CAD build for the part. Positions are in the model's coordinates, mm. Coordinates: 2 decimals unless noted, no trailing zeros. Order: outer loops, then holes, each group sorted by start corner. A loop starts at its lowest first (then second) coordinate and runs counter-clockwise, first axis right, second up. Notation, with made-up numbers: M -3,33.5 L 19,33.5 A13 cw 19,42.5 Z; hole C 62,29 d1. An arc over 180 degrees is marked long. Write item = value, one per line. Start each with the question number.
```python
from build123d import *

# Parameters (mm, degrees)
SKETCH7_R           = 24
SKETCH7_R_2         = 20.5
BOSS_EXTRUDE6_DEPTH = 3.5
FILLET4_R           = 1.75


with BuildPart() as part:
    # Sketch7 → Boss-Extrude6 (new body)
    with BuildSketch(Plane(origin=(-0.280788986, 0.442554621, -13.906554041), x_dir=(-1, 0, 0), z_dir=(0, 0, -1))):
        with Locations((-13.807967582, -75.62783073)):
            Circle(SKETCH7_R)
        with Locations((-13.807967582, -75.62783073)):
            Circle(SKETCH7_R_2, mode=Mode.SUBTRACT)
    extrude(amount=BOSS_EXTRUDE6_DEPTH)

    # Fillet4
    fillet4_edges = [part.edges().sort_by_distance(p)[0] for p in [
        (37.527178596, -75.18527611, -13.906554041),
        (37.527178596, -75.18527611, -17.406554041),
        (34.027178596, -75.18527611, -13.906554041),
        (34.027178596, -75.18527611, -17.406554041),
    ]]
    fillet(fillet4_edges, radius=FILLET4_R - 0.0001)  # a hair under: the kernel refuses the full size


solid = part.part
```
1. Flat gauge pins, fed straight in: pin 1 (1 mm diameter, centred on y = -75.5, z = -17, fed in from -X); pin 2 (2 mm diameter, centred on x = 19.5, z = -17, fed in from -Y); pin 3 (1.5 mm diameter, centred on y = -86, z = -16, fed in from -X). Where does each tip first touch, or does it go through?
2. Slice it at A-A (z = -14.8). Write the cut outline in (x, y).
3. Probe L1, parallel to Y at x = 19, z = -15.25; L2, parallel to Y at x = -3.5, z = -15.2; L3, parallel to X at y = -88, z = -15.45. List the from-to ranges inside material, lowest first.
Calculated:
q1.pin_1 = -10.25
q1.pin_2 = -98.49
q1.pin_3 = -8.24
q2.outline = C 13.53,-75.19 d47.55; hole C 13.53,-75.19 d41.45
q3.L1 = -98.5 to -94.99, -55.38 to -51.87
q3.L2 = -92.01 to -86.71, -63.66 to -58.36
q3.L3 = -6.75 to -2.49, 29.54 to 33.81
